Source: CAD feature listing. Evaluate the final solid. Frame: model axes, mm. A direction names the side the tool comes from. Coordinates: 2 decimals unless noted, no trailing zeros. Order: outer loops, then holes, each group sorted by start corner. A loop starts at its lowest first (then second) coordinate and runs counter-clockwise, first axis right, second up.
```python
from build123d import *

# Parameters (mm, degrees)
SKETCH1_W             = 192.532
SKETCH1_H             = 157.48
BASE_DEPTH            = 5.334
CENTER_CUT_DEPTH      = 249.791022708
CENTER_CUT_DEPTH_BACK = 249.791022708
FILLET1_R             = 6.35
CUT_EXTRUDE3_DEPTH    = 249.791022708


with BuildPart() as part:
    # Sketch1 → Base (new body)
    with BuildSketch(Plane(origin=(0, 0, 0), x_dir=(1, 0, 0), z_dir=(0, 1, 0))):
        with Locations((96.266, 78.74)):
            Rectangle(SKETCH1_W, SKETCH1_H)
    extrude(amount=BASE_DEPTH)

    # Sketch2 → Center Cut (cut, two sides: drawn at the far end of the back side and taken through both)
    with BuildSketch(Plane(origin=(0, 5.334, 0), x_dir=(1, 0, 0), z_dir=(0, 1, 0)).offset(-CENTER_CUT_DEPTH_BACK)):
        with BuildLine():
            Line((217.68055776, 642.475883119), (178.816, 157.48))
            Line((178.816, 157.48), (172.200955719, 74.93))
            ThreePointArc((172.200955719, 74.93), (96.266, 5.08), (20.331044281, 74.93))
            Line((20.331044281, 74.93), (13.716, 157.48))
            Line((13.716, 157.48), (-25.14855776, 642.475883119))
            Line((-25.14855776, 642.475883119), (-25.14855776, 1615.577029953))
            Line((-25.14855776, 1615.577029953), (217.68055776, 1615.577029953))
            Line((217.68055776, 1615.577029953), (217.68055776, 642.475883119))
        make_face()
    extrude(amount=CENTER_CUT_DEPTH + CENTER_CUT_DEPTH_BACK, mode=Mode.SUBTRACT)

    # Fillet1
    fillet1_edges = [part.edges().sort_by_distance(p)[0] for p in [
        (178.816, 2.667, -157.48),
        (13.716, 2.667, -157.48),
    ]]
    fillet(fillet1_edges, radius=FILLET1_R)

    # Sketch7 → Cut-Extrude3 (cut, through all)
    with BuildSketch(Plane(origin=(0, 5.334, 0), x_dir=(1, 0, 0), z_dir=(0, 1, 0))):
        with BuildLine():
            Line((6.35, 40.9102037), (24.260569325, 40.9102037))
            ThreePointArc((24.260569325, 40.9102037), (35.834123486, 25.043972393), (50.827976512, 12.360564994))
            Line((50.827976512, 12.360564994), (50.827976512, 0))
            Line((50.827976512, 0), (6.35, 0))
            Line((6.35, 0), (6.35, 40.9102037))
        make_face()
        with BuildLine():
            Line((186.182, 40.9102037), (186.182, 0))
            Line((186.182, 0), (141.704023488, 0))
            Line((141.704023488, 0), (141.704023488, 12.360564994))
            ThreePointArc((141.704023488, 12.360564994), (156.697876514, 25.043972393), (168.271430675, 40.9102037))
            Line((168.271430675, 40.9102037), (186.182, 40.9102037))
        make_face()
    extrude(amount=-CUT_EXTRUDE3_DEPTH, mode=Mode.SUBTRACT)


solid = part.part
```
1. Section query A-A on z = -122.5. Return loops of the section in (x, y), plus the area to 3 significant figures.
Findings:
outline: (0, 0) - (16.52, 0) - (16.52, 5.33) - (0, 5.33) - close; (176.01, 0) - (192.53, 0) - (192.53, 5.33) - (176.01, 5.33) - close
area: 176 mm2
2. Section query C-C on y = 4.3. Return loops of the section in (x, z).
Findings:
outline: (0, -157.48) - (7.85, -157.48) arc R6.35 ccw to (14.18, -151.64) - (20.33, -74.93) arc R76.2 cw to (172.2, -74.93) - (178.35, -151.64) arc R6.35 ccw to (184.68, -157.48) - (192.53, -157.48) - (192.53, 0) - (186.18, 0) - (186.18, -40.91) - (168.27, -40.91) arc R82.55 ccw to (141.7, -12.36) - (141.7, 0) - (50.83, 0) - (50.83, -12.36) arc R82.55 ccw to (24.26, -40.91) - (6.35, -40.91) - (6.35, 0) - (0, 0) - close
3. Access query for faces 5 (the face through (189, 3, -157.48)), 6 (the face through (175.317, 2.63, -113.821)), 7 (the face through (15, 3, -40.91)). Directions: +Z, -Z, +X, -X, +Y, -Y. A direction counts if a zero-diameter tool reaches every point of the face in a straight line with its end or side. Return the directions, or none.
Findings:
face 5: -Z, +X, -X, +Y, -Y
face 6: -Z, +Y, -Y
face 7: +Z, +Y, -Y
4. Section query D-D on z = -78. Return loops of the section in (x, y), plus the area to 3 significant figures.
Findings:
outline: (0, 0) - (20.09, 0) - (20.09, 5.33) - (0, 5.33) - close; (172.45, 0) - (192.53, 0) - (192.53, 5.33) - (172.45, 5.33) - close
area: 214 mm2
5. Pin query (flat end, axial travel): P1, Ø2.5, axis at x = 180.5, y = 1.5, coming from the +Z side; P2, Ø3, axis at x = 160.5, y = 3.5, coming from the -Z side. Return the tip coordinate at first contact, or that it passes through.
Findings:
P1: stops at z = -40.91
P2: stops at z = -42.74
6. Section query B-B on z = -9.5. Return loops of the section in (x, y).
Findings:
outline: (0, 0) - (6.35, 0) - (6.35, 5.33) - (0, 5.33) - close; (50.83, 0) - (70.69, 0) - (70.69, 5.33) - (50.83, 5.33) - close; (121.84, 0) - (141.7, 0) - (141.7, 5.33) - (121.84, 5.33) - close; (186.18, 0) - (192.53, 0) - (192.53, 5.33) - (186.18, 5.33) - close
7. Ray query, line 1 (X direction, y = 1.5, z = -106.5); line 2 (Z direction, x = 96, y = 0.8); line 3 (X direction, y = 1.65, z = -67.5). Return the intervals inside material, ascending.
Findings:
line 1: x = 0 to 17.8, 174.73 to 192.53
line 2: z = -5.08 to 0
line 3: x = 0 to 21.32, 171.21 to 192.53
8. Draft query along X for faces 1 (the face through (0, 3, -78)), 2 (the face through (192.532, 3, -78)), 3 (the face through (189, 3, 0)), 4 (the face through (35.647, 2.704, -25.246)). Return one class per face: released by +X, released by -X, zero draft, split by the parting line, or undercut.
Findings:
face 1: released by -X
face 2: released by +X
face 3: zero draft
face 4: undercut
